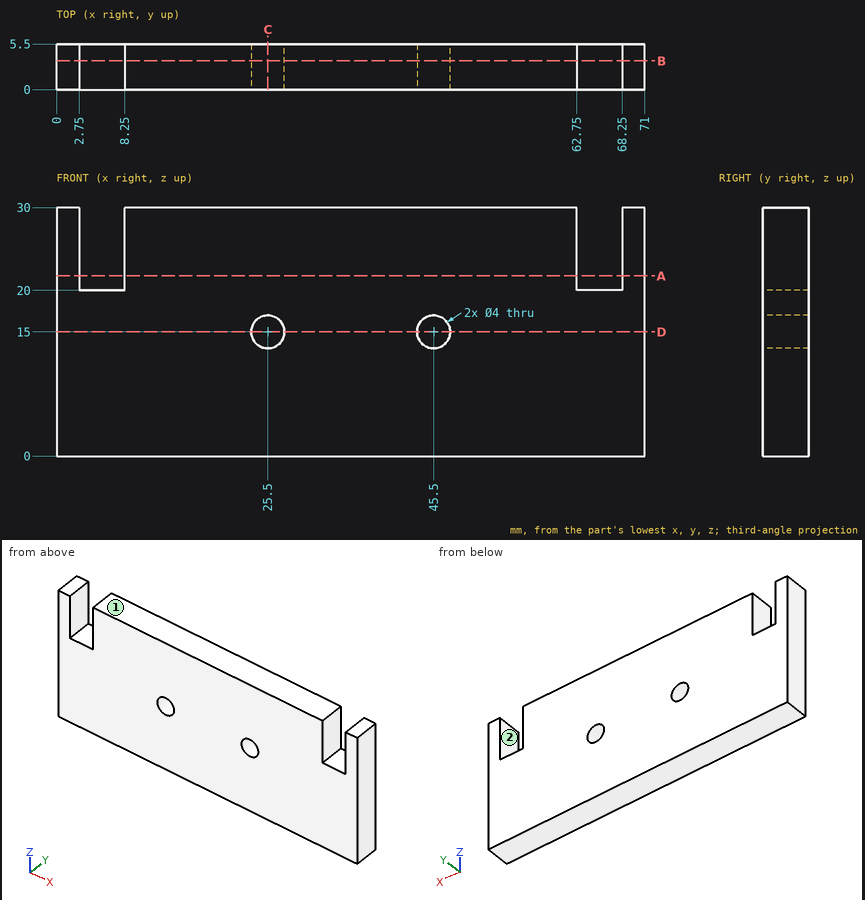
Geometry: see drawing. Coordinates: mm, zero at the bounding-box minimum. A direction names the side the tool comes from. Round coordinates to 2 decimals unless told otherwise and drop trailing zeros. Write each loop counter-clockwise with the first axis right and the second up, starting at its lowest first coordinate (ties: lowest second). Pieces come first, ordered by that corner, then holes.
1) Cut plane B-B (y = 3.45). Return the cut outline in (x, z).
2) Cut plane C-C (x = 25.5). Return the cut outline in (y, z).
3) Cut plane D-D (z = 15). Return the cut outline in (x, y).
4) Cut plane A-A (z = 21.75). Return the cut outline in (x, y), then the cut area to 3 significant figures.
5) Ray query, L1, parallel to X at y = 4, z = 15; L2, parallel to X at y = 4.3, z = 25; L3, parallel to Z at x = 45.5, y = 1.65. Return the intervals inside material, ascending.
6) Reachability of the marked faces 1 and 2 from +Z, -Z, +X, -X, +Y, -Y: full face, straight path, thin tool, end or side. Return the list, or none.
7) Contact query for a flat-ended pin moving along its axis: P1, Ø1.6, axis at x = 65.5, y = 3, coming from the +Z side. Output: stop coordinate, or through.
Geometry says:
1. outline: (0, 0) - (71, 0) - (71, 30) - (68.25, 30) - (68.25, 20) - (62.75, 20) - (62.75, 30) - (8.25, 30) - (8.25, 20) - (2.75, 20) - (2.75, 30) - (0, 30) - close; hole circle Ø4 at (25.5, 15); hole circle Ø4 at (45.5, 15)
2. outline: (0, 0) - (5.5, 0) - (5.5, 13) - (0, 13) - close; (0, 17) - (5.5, 17) - (5.5, 30) - (0, 30) - close
3. outline: (0, 0) - (23.5, 0) - (23.5, 5.5) - (0, 5.5) - close; (27.5, 0) - (43.5, 0) - (43.5, 5.5) - (27.5, 5.5) - close; (47.5, 0) - (71, 0) - (71, 5.5) - (47.5, 5.5) - close
4. outline: (0, 0) - (2.75, 0) - (2.75, 5.5) - (0, 5.5) - close; (8.25, 0) - (62.75, 0) - (62.75, 5.5) - (8.25, 5.5) - close; (68.25, 0) - (71, 0) - (71, 5.5) - (68.25, 5.5) - close
4. area: 330 mm2
5. L1: x = 0 to 23.5, 27.5 to 43.5, 47.5 to 71
5. L2: x = 0 to 2.75, 8.25 to 62.75, 68.25 to 71
5. L3: z = 0 to 13, 17 to 30
6. face 1: +Z, +X, -X, +Y, -Y
6. face 2: +Z, +Y, -Y
7. P1: stops at z = 20
